For this review, take the finished solid that the model builds, in its own axes (mm). A direction names the side the tool comes from. Round coordinates to 2 decimals unless told otherwise and drop trailing zeros. Order: outer loops, then holes, each group sorted by start corner. A loop starts at its lowest first (then second) coordinate and runs counter-clockwise, first axis right, second up. Notation, with made-up numbers: M 5,63 L 59,63 A20 cw 59,82 Z; hole C -16,-25.5 d3. An arc over 180 degrees is marked long. Use a Markdown table: item, result.
from build123d import *

# Parameters (mm, degrees)
BOSS_EXTRUDE1_DEPTH = 25
SKETCH2_R           = 11
SKETCH2_R_2         = 9
BOSS_EXTRUDE2_DEPTH = 200
CIRPATTERN1_COUNT   = 4


with BuildPart() as part:
    # Sketch1 → Boss-Extrude1 (new body)
    with BuildSketch(Plane(origin=(0, 0, 0), x_dir=(1, 0, 0), z_dir=(0, 1, 0))):
        Polygon((-75, 31.066017178), (-75, -31.066017178), (-31.066017178, -75), (31.066017178, -75), (75, -31.066017178), (75, 31.066017178), (31.066017178, 75), (-31.066017178, 75), align=None)
    extrude(amount=BOSS_EXTRUDE1_DEPTH)

    # Sketch2 → Boss-Extrude2 (add)
    with BuildSketch(Plane.ZY.offset(75)):
        with Locations(Location((0, 12.5, 0), (0, 0, 180))):
            Circle(SKETCH2_R)
        with Locations((0, 12.5)):
            Circle(SKETCH2_R_2, mode=Mode.SUBTRACT)
    boss_extrude2 = extrude(amount=BOSS_EXTRUDE2_DEPTH)

    # CirPattern1: Boss-Extrude2 ×4 about axis
    cirpattern1_axis = Axis((0, 0, 0), (0, 1, 0))
    for i in range(1, CIRPATTERN1_COUNT):
        add(boss_extrude2.rotate(cirpattern1_axis, i * 360 / CIRPATTERN1_COUNT))


solid = part.part
Q1. Machinability: for faces 4 (the flat face through (75, 12, 0)), 5 (the flat face through (-1, 0, -1)), 6 (the cylindrical face through (2.38, 23.24, 173.6)), 7 (the flat face through (0, 12, -75)), which of the approach directions +Z, -Z, +X, -X, +Y, -Y give a long, thin tool a straight path to every point of the face, cutting with its end or side? Answer none if there is none.
Determined:
| item | result |
|---|---|
| face 4 | +X |
| face 5 | +Z, -Z, +X, -X, -Y |
| face 6 | +Z |
| face 7 | -Z |
Q2. Add section B-B (z = 0). Write out the cut boundary in (x, y).
Determined:
| item | result |
|---|---|
| outline | M -275,1.5 L -75,1.5 L -75,0 L 75,0 L 75,1.5 L 275,1.5 L 275,3.5 L 75,3.5 L 75,21.5 L 275,21.5 L 275,23.5 L 75,23.5 L 75,25 L -75,25 L -75,23.5 L -275,23.5 L -275,21.5 L -75,21.5 L -75,3.5 L -275,3.5 Z |
Q3. Add section C-C (x = -92). Write out the cut boundary in (y, z), then the cut area to 3 significant figures.
Determined:
| item | result |
|---|---|
| outline | C 12.5,0 d22; hole C 12.5,0 d18 |
| area | 126 mm^2 |
Q4. Draft analysis for pull direction X (two halves, no side actions). For faces 1 (the cylindrical face through (-173.6, 7.02, -7.14)), 2 (the cylindrical face through (-1.951, 3.714, 173.6)), 3 (the flat face through (53.341, 12.325, -52.725)), state which applies: pulls with the +X half, pulls with the -X half, needs draft (parallel to the pull), parting line crosses it, or undercut.
Determined:
| item | result |
|---|---|
| face 1 | needs draft |
| face 2 | undercut |
| face 3 | pulls with the +X half |
Q5. Clearance check with flat-ended pins moving along their axes: pin 1 (10 mm diameter, centred on y = 6.5, z = 74, fed in from -X); pin 2 (9 mm diameter, centred on x = 3.5, y = 12, fed in from +Z); pin 3 (1.5 mm diameter, centred on y = 14, z = 27, fed in from +X). State where each tip first meets the part, or that it passes through.
Determined:
| item | result |
|---|---|
| pin 1 | stops at x = -37.07 |
| pin 2 | stops at z = 75 |
| pin 3 | stops at x = 75 |
Q6. Add section A-A (x = 0). Write out the cut boundary in (y, z), then the cut area to 3 significant figures.
Determined:
| item | result |
|---|---|
| outline | M 0,-75 L 1.5,-75 L 1.5,-275 L 3.5,-275 L 3.5,-75 L 21.5,-75 L 21.5,-275 L 23.5,-275 L 23.5,-75 L 25,-75 L 25,75 L 23.5,75 L 23.5,275 L 21.5,275 L 21.5,75 L 3.5,75 L 3.5,275 L 1.5,275 L 1.5,75 L 0,75 Z |
| area | 5,350 mm^2 |
Q7. Wall thickness on line 1 along X through (y, z) = (11, 96); line 2 along Y through (x, z) = (0, -120); line 3 along X through (y, z) = (12.25, -136.5): over which ranges is each line inside the solid? List them lowest first. Write a range as [from, to].
Determined:
| item | result |
|---|---|
| line 1 | x = [-10.9, -8.87], [8.87, 10.9] |
| line 2 | y = [1.5, 3.5], [21.5, 23.5] |
| line 3 | x = [-11, -9], [9, 11] |
Q8. Add section D-D (z = 150). Write out the cut boundary in (x, y).
Determined:
| item | result |
|---|---|
| outline | C 0,12.5 d22; hole C 0,12.5 d18 |
